from build123d import *

# Parameters (mm, degrees)
SKETCH1_R           = 26.5
BOSS_EXTRUDE1_DEPTH = 32
SKETCH2_R           = 20
BOSS_EXTRUDE2_DEPTH = 7
SKETCH3_R           = 18.5
BOSS_EXTRUDE3_DEPTH = 1
SKETCH4_R           = 1.25
CUT_EXTRUDE1_DEPTH  = 3
SKETCH5_R           = 1.5
CUT_EXTRUDE2_DEPTH  = 4
CUT_EXTRUDE3_START  = -5
SKETCH6_R           = 1.25
CUT_EXTRUDE3_DEPTH  = 5
SKETCH7_W           = 60.119067385
SKETCH7_H           = 14
CUT_EXTRUDE4_DEPTH  = 3


with BuildPart() as part:
    # Sketch1 → Boss-Extrude1 (new body)
    with BuildSketch(Plane(origin=(0, 0, 0), x_dir=(1, 0, 0), z_dir=(0, 1, 0))):
        with Locations(Location((0, 0, 0), (0, 0, 270))):
            Circle(SKETCH1_R)
    extrude(amount=BOSS_EXTRUDE1_DEPTH)

    # Sketch2 → Boss-Extrude2 (add)
    with BuildSketch(Plane.XZ):
        with Locations(Location((0, 0, 0), (0, 0, 270))):
            Circle(SKETCH2_R)
    extrude(amount=BOSS_EXTRUDE2_DEPTH)

    # Sketch3 → Boss-Extrude3 (add)
    with BuildSketch(Plane(origin=(0, 32, 0), x_dir=(1, 0, 0), z_dir=(0, 1, 0))):
        with Locations(Location((0, 0, 0), (0, 0, 270))):
            Circle(SKETCH3_R)
    extrude(amount=BOSS_EXTRUDE3_DEPTH)

    # Sketch4 → Cut-Extrude1 (cut)
    with BuildSketch(Plane.XZ):
        with Locations(Location((0, 23.75, 0), (0, 0, 270))):
            Circle(SKETCH4_R)
        with Locations(Location((20.56810334, 11.875, 0), (0, 0, 270))):
            Circle(SKETCH4_R)
        with Locations(Location((20.56810334, -11.875, 0), (0, 0, 270))):
            Circle(SKETCH4_R)
        with Locations(Location((0, -23.75, 0), (0, 0, 270))):
            Circle(SKETCH4_R)
        with Locations(Location((-20.56810334, -11.875, 0), (0, 0, 270))):
            Circle(SKETCH4_R)
        with Locations(Location((-20.56810334, 11.875, 0), (0, 0, 270))):
            Circle(SKETCH4_R)
    extrude(amount=-CUT_EXTRUDE1_DEPTH, mode=Mode.SUBTRACT)

    # Sketch5 → Cut-Extrude2 (cut)
    with BuildSketch(Plane(origin=(0, 33, 0), x_dir=(1, 0, 0), z_dir=(0, 1, 0))):
        with Locations(Location((0, 13.5, 0), (0, 0, 270))):
            Circle(SKETCH5_R)
        with Locations(Location((11.691342951, -6.75, 0), (0, 0, 270))):
            Circle(SKETCH5_R)
        with Locations(Location((-11.691342951, -6.75, 0), (0, 0, 270))):
            Circle(SKETCH5_R)
    extrude(amount=-CUT_EXTRUDE2_DEPTH, mode=Mode.SUBTRACT)

    # Sketch6 → Cut-Extrude3 (cut)
    with BuildSketch(Plane(origin=(0, 32, 0), x_dir=(1, 0, 0), z_dir=(0, 1, 0)).offset(CUT_EXTRUDE3_START)):
        with Locations(Location((0, 23.75, 0), (0, 0, 90))):
            Circle(SKETCH6_R)
        with Locations(Location((20.56810334, -11.875, 0), (0, 0, 90))):
            Circle(SKETCH6_R)
        with Locations(Location((-20.56810334, -11.875, 0), (0, 0, 90))):
            Circle(SKETCH6_R)
    extrude(amount=CUT_EXTRUDE3_DEPTH, mode=Mode.SUBTRACT)

    # Sketch7 → Cut-Extrude4 (cut)
    with BuildSketch(Plane.XZ):
        with Locations((1.148519733, 0)):
            Rectangle(SKETCH7_W, SKETCH7_H)
    extrude(amount=-CUT_EXTRUDE4_DEPTH, mode=Mode.SUBTRACT)


solid = part.part
Check sheet for the modelled part. Datum: model origin and axes. Units: mm. A direction names the side the tool comes from. Round coordinates to 2 decimals unless told otherwise and drop trailing zeros. Loops run counter-clockwise (first coordinate to the right, second up) from the corner with the lowest first, then second, coordinate; pieces in that order, holes last. Notation, with made-up numbers: (-36.75, -39.5) -> (12.25, -39.5) arc R25 ccw to (12.25, -1.5) -> close; hole circle Ø1 at (55, 72.25). An arc over 180 degrees is marked (long way). Put each result on its own line as item: value. Start each with the question number.
1. Section check D-D (y = 12.5). Enter the section's corners in (x, z).
2. Access from +Z, -Z, +X, -X, +Y, -Y to the whole of each face (thin tool, end or side, straight path). Record for faces 5 (the face through (18, 32, 6)), 6 (the face through (-19.723, 1.479, -10.954)), 7 (the face through (0, 3, 0)).
3. Gauge pin test, flat ends, axial feed: pin 1 (2 mm diameter, centred on x = 20.57, z = 11.88, fed in from -Y); pin 2 (2 mm diameter, centred on x = 21, z = 12, fed in from -Y); pin 3 (2.5 mm diameter, centred on x = 0, z = -13.5, fed in from +Y); pin 4 (5 mm diameter, centred on x = 11.69, z = 6.75, fed in from +Y). Record the tip position at first contact, or that the pin passes through.
4. Section check C-C (z = 15.5). Enter the section's corners in (x, y).
5. Section check B-B (z = 0). Enter the section's corners in (x, y).
6. Section check A-A (y = 2). Enter the section's corners in (x, z) (3 decimals), plus the area to 3 significant figures.
7. Draft check along X on faces 1 (the face through (-0.479, 1.479, 22.595)), 2 (the face through (0, 27, -24)), 3 (the face through (0, 0, 21)), 4 (the face through (-7.086, 32.493, 17.089)). Enter one of: +X half, -X half, draft (parallel to the pull), parting line (faces both ways), or undercut.
8. Scan lines: probe 1 along Y at (x, z) = (-12.5, 0); probe 2 along Z at (x, y) = (-20, 2.5); probe 3 along Z at (x, y) = (-21, 1). Record each from-to range of solid material in increasing order.
Findings:
1. outline: circle Ø53 at (0, 0)
2. face 5: +Y
2. face 6: -Y
2. face 7: +X, -X
3. pin 1: stops at y = 3
3. pin 2: stops at y = 0
3. pin 3: stops at y = 29
3. pin 4: stops at y = 33
4. outline: (-21.49, 0) -> (-12.64, 0) -> (-12.64, -7) -> (12.64, -7) -> (12.64, 0) -> (21.49, 0) -> (21.49, 32) -> (10.1, 32) -> (10.1, 33) -> (-10.1, 33) -> (-10.1, 32) -> (-21.49, 32) -> close
5. outline: (-26.5, 3) -> (26.5, 3) -> (26.5, 32) -> (18.5, 32) -> (18.5, 33) -> (-18.5, 33) -> (-18.5, 32) -> (-26.5, 32) -> close; (-20, -7) -> (20, -7) -> (20, 0) -> (-20, 0) -> close
6. outline: (-25.559, -7) arc R26.5 ccw to (25.559, -7) -> close; (-25.559, 7) -> (25.559, 7) arc R26.5 ccw to start; hole circle Ø2.5 at (-20.568, -11.875); hole circle Ø2.5 at (-20.568, 11.875); hole circle Ø2.5 at (0, -23.75); hole circle Ø2.5 at (0, 23.75); hole circle Ø2.5 at (20.568, -11.875); hole circle Ø2.5 at (20.568, 11.875)
6. area: 1,440 mm^2
7. face 1: undercut
7. face 2: undercut
7. face 3: draft
7. face 4: parting line
8. probe 1: y = -7 to 0, 3 to 33
8. probe 2: z = -17.39 to -12.99, -10.76 to -7, 7 to 10.76, 12.99 to 17.39
8. probe 3: z = -16.16 to -13.05, -10.7 to -7, 7 to 10.7, 13.05 to 16.16
